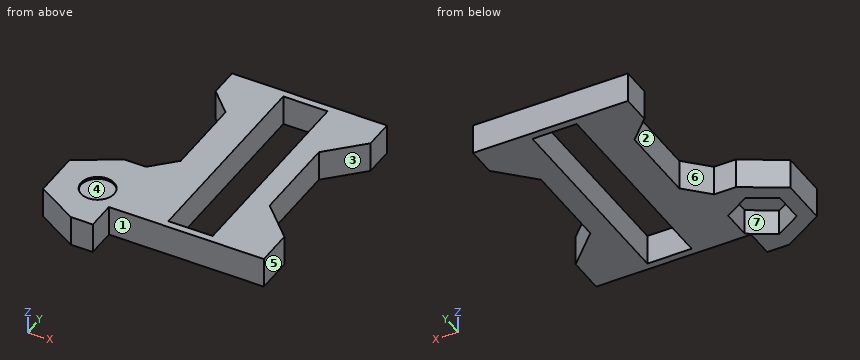
from build123d import *

# Parameters (mm, degrees)
SKETCH_R        = 2.25
SKETCH_W        = 6
SKETCH_H        = 28
PAD_DEPTH       = 4.1
POCKET_DEPTH    = 3.5
SKETCH003_W     = 21
SKETCH003_H     = 4.1
POCKET001_DEPTH = 1
SKETCH002_R     = 2.25
PAD001_DEPTH    = 0.3


with BuildPart() as part:
    # Sketch → Pad (new body)
    with BuildSketch(Plane.XY):
        Polygon((-10.5, 15.5), (10.5, 15.5), (10.5, 10.491002), (6, 5.991002), (6, -5.991002), (10.5, -10.491002), (10.5, -15.5), (-10.5, -15.5), (-10.5, -17.717136), (-10.5, -19.420319), (-13.45, -19.420319), (-19.053461, -16.18516), (-19.053461, -9.71484), (-13.45, -6.479681), (-10.508209, -6.479681), (-7.472105, -3.443576), (-7.472105, 7.463107), (-10.5, 10.491002), align=None)
        with Locations((-13.45, -12.95)):
            Circle(SKETCH_R, mode=Mode.SUBTRACT)
        with Locations((0, -0.5)):
            Rectangle(SKETCH_W, SKETCH_H, mode=Mode.SUBTRACT)
    extrude(amount=PAD_DEPTH)

    # Sketch001 → Pocket (cut)
    with BuildSketch(Plane(origin=(0, 0, 0), x_dir=(1, 0, 0), z_dir=(0, 0, -1))):
        Polygon((-13.45, 8.879681), (-9.925, 10.91484), (-9.925, 14.98516), (-13.45, 17.020319), (-16.975, 14.98516), (-16.975, 10.91484), align=None)
    extrude(amount=-POCKET_DEPTH, mode=Mode.SUBTRACT)

    # Sketch003 → Pocket001 (cut)
    with BuildSketch(Plane(origin=(0, 15.5, 0), x_dir=(-1, 0, 0), z_dir=(0, 1, 0))):
        with Locations((0, 2.05)):
            Rectangle(SKETCH003_W, SKETCH003_H)
    extrude(amount=-POCKET001_DEPTH, mode=Mode.SUBTRACT)

    # Sketch002 → Pad001 (new body)
    with BuildSketch(Plane(origin=(0, 0, 3.5), x_dir=(1, 0, 0), z_dir=(0, 0, -1))):
        with Locations((-13.45, 12.95)):
            Circle(SKETCH002_R)
    extrude(amount=-PAD001_DEPTH)


solid = part.part
Geometry: final body of the model. Coordinates: model frame, mm. Face numbers are marked on the shaded views. A direction names the side the tool comes from. Give positions to 0.01 mm unless a question says otherwise; leave off trailing zeros. Order: outer loops, then holes, each group sorted by start corner. A loop starts at its lowest first (then second) coordinate and runs counter-clockwise, first axis right, second up. Notation, with made-up numbers: (-20, 58) -> (15, 58) arc R15 ccw to (15, 74) -> close; hole circle Ø9 at (4.5, 7.25). An arc over 180 degrees is marked (long way). Put each result on its own line as item: value.
Q1. Section A-A, the plane y = -12.95. Return loops of the section in (x, z) (3 decimals).
Here are the results:
outline: (-19.053, 0) -> (-16.975, 0) -> (-16.975, 3.5) -> (-9.925, 3.5) -> (-9.925, 0) -> (-3, 0) -> (-3, 4.1) -> (-11.2, 4.1) -> (-11.2, 3.8) -> (-15.7, 3.8) -> (-15.7, 4.1) -> (-19.053, 4.1) -> close; (3, 0) -> (10.5, 0) -> (10.5, 4.1) -> (3, 4.1) -> close
Q2. Section C-C, the plane y = 2. Return loops of the section in (x, z).
Here are the results:
outline: (-7.47, 0) -> (-3, 0) -> (-3, 4.1) -> (-7.47, 4.1) -> close; (3, 0) -> (6, 0) -> (6, 4.1) -> (3, 4.1) -> close
Q3. Reachability of the marked faces 1, 2, 3 and 4 from +Z, -Z, +X, -X, +Y, -Y: full face, straight path, thin tool, end or side. Return the list, or none.
Here are the results:
face 1: +Z, -Z, +X, -Y
face 2: +Z, -Z, -X
face 3: +Z, -Z, +X
face 4: +Z
Q4. Draft query along X for the marked faces 5, 6 and 7. Return one class per face: released by +X, released by -X, zero draft, split by the parting line, or undercut.
Here are the results:
face 5: released by +X
face 6: released by -X
face 7: undercut
Q5. Section B-B, the plane z = 1.45. Return loops of the section in (x, y) (3 decimals), then the cut area to 3 significant figures.
Here are the results:
outline: (-19.053, -16.185) -> (-13.45, -19.42) -> (-10.5, -19.42) -> (-10.5, -15.5) -> (10.5, -15.5) -> (10.5, -10.491) -> (6, -5.991) -> (6, 5.991) -> (10.5, 10.491) -> (10.5, 14.5) -> (-10.5, 14.5) -> (-10.5, 10.491) -> (-7.472, 7.463) -> (-7.472, -3.444) -> (-10.508, -6.48) -> (-13.45, -6.48) -> (-19.053, -9.715) -> close; hole (-16.975, -14.985) -> (-13.45, -17.02) -> (-9.925, -14.985) -> (-9.925, -10.915) -> (-13.45, -8.88) -> (-16.975, -10.915) -> close; hole (-3, -14.5) -> (3, -14.5) -> (3, 13.5) -> (-3, 13.5) -> close
area: 395 mm^2
Q6. Pin query (flat end, axial travel): pin 1 (6 mm diameter, centred on x = 1.5, y = 6, fed in from +Z); pin 2 (1.2 mm diameter, centred on y = 13, z = 3, fed in from -X); pin 3 (2 mm diameter, centred on x = 1, z = 1.5, fed in from -Y); pin 4 (2 mm diameter, centred on x = -14, y = -14.5, fed in from -Z). Return the tip coordinate at first contact, or that it passes through.
Here are the results:
pin 1: stops at z = 4.1
pin 2: stops at x = -10.5
pin 3: stops at y = -15.5
pin 4: stops at z = 3.5
Q7. Material intervals for L1, parallel to X at y = -12.95, z = 3.95; L2, parallel to Y at x = -13.45, z = 4; L3, parallel to X at y = 2, z = 1.85, sorted ascending.
Here are the results:
L1: x = -19.05 to -15.7, -11.2 to -3, 3 to 10.5
L2: y = -19.42 to -15.2, -10.7 to -6.48
L3: x = -7.47 to -3, 3 to 6
Q8. Section D-D, the plane x = -6.5. Return loops of the section in (y, z), then the cut area to 3 significant figures.
Here are the results:
outline: (-15.5, 0) -> (14.5, 0) -> (14.5, 4.1) -> (-15.5, 4.1) -> close
area: 123 mm^2
